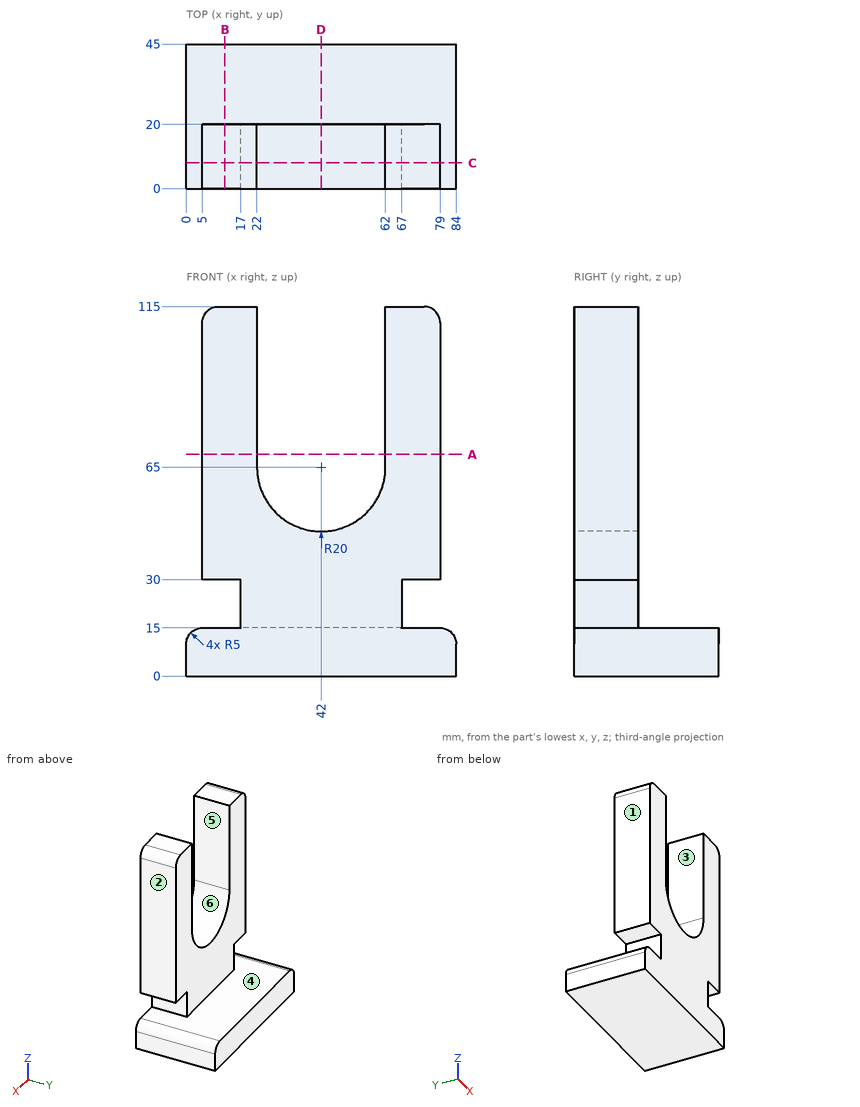
For this review, use the dimensioned drawing (mm, ordinates from the lowest corner) and the shaded views. A direction names the side the tool comes from. Give positions to 0.01 mm unless a question says otherwise; leave off trailing zeros. Write each loop counter-clockwise with the first axis right and the second up, starting at its lowest first coordinate (ties: lowest second). Pieces come first, ordered by that corner, then holes. Notation, with made-up numbers: M 55.5,30.5 L 112.5,30.5 A28 ccw 112.5,54.5 Z; hole C 38.5,59.25 d10. An arc over 180 degrees is marked long. Answer as a JSON object with one key per item and string values. Group by question number.
Item 1: Consider section A-A on z = 69. Write out the cut boundary in (x, y).
Item 2: Draft analysis for pull direction Z (two halves, no side actions). For the marked faces 4, 5 and 6, state which applies: +Z half, -Z half, draft (parallel to the pull), parting line (faces both ways), or undercut.
Item 3: For probe 1 along Z at (x, y) = (74, 17); probe 2 along X at (y, z) = (9.5, 97); probe 3 along X at (y, z) = (7, 17.5), list the stretches that pass through material, from the lowest coordinate up. Write a range as [from, to].
Item 4: Consider section C-C on y = 8. Write out the cut boundary in (x, z).
Item 5: Consider section D-D on x = 42. Write out the cut boundary in (y, z), plus the area to 4 significant figures.
Item 6: Tool access review of the marked faces 1, 2 and 3: name each direction out of +Z, -Z, +X, -X, +Y, -Y from which nothing blocks a thin tool from reaching the whole face with its end or side.
Item 7: For pin 1 Ø22 at (x, z) = (24, 51.5) entering from +Y; pin 2 Ø1 at (y, z) = (5, 33) entering from -X; pin 3 Ø10 at (y, z) = (22, 22.5) entering from -X; pin 4 Ø9.5 at (x, y) = (13.5, 13.5) entering from -Z, all flat-tipped, find the tip position at first contact; note any pin that passes through.
Item 8: Consider section B-B on x = 12. Write out the cut boundary in (y, z), plus the area to 4 significant figures.
Check result:
{
 "1": {"outline": "M 5,0 L 22,0 L 22,20 L 5,20 Z; M 62,0 L 79,0 L 79,20 L 62,20 Z"},
 "2": {"face 4": "undercut", "face 5": "draft", "face 6": "+Z half"},
 "3": {"probe 1": "z = [0, 15], [30, 115]", "probe 2": "x = [5, 22], [62, 79]", "probe 3": "x = [17, 67]"},
 "4": {"outline": "M 0,0 L 84,0 L 84,10 A5 ccw 79,15 L 67,15 L 67,30 L 79,30 L 79,110 A5 ccw 74,115 L 62,115 L 62,65 A20 cw 22,65 L 22,115 L 10,115 A5 ccw 5,110 L 5,30 L 17,30 L 17,15 L 5,15 A5 ccw 0,10 Z"},
 "5": {"outline": "M 0,0 L 45,0 L 45,15 L 20,15 L 20,45 L 0,45 Z", "area": "1,275 mm^2"},
 "6": {"face 1": "+Z, -X, +Y, -Y", "face 2": "+Z, +X, +Y, -Y", "face 3": "+Z, +Y, -Y"},
 "7": {"pin 1": "stops at y = 20", "pin 2": "stops at x = 5", "pin 3": "stops at x = 17", "pin 4": "stops at z = 0"},
 "8": {"outline": "M 0,0 L 45,0 L 45,15 L 0,15 Z; M 0,30 L 20,30 L 20,115 L 0,115 Z", "area": "2,375 mm^2"}
}
